from build123d import *

# Parameters (mm, degrees)
F0_W            = 307.8816831112
F0_H            = 200.2553716302
F1_DEPTH        = 25.4
F2_W            = 307.8816831112
F2_H            = 25.4
F3_DEPTH        = 174.76264
F4_DEPTH        = 949.00905
F5_W            = 1324.0270616302
F5_H            = 25.4
F6_DEPTH        = 25.4
F7_W            = 25.4
F7_H            = 1324.0270616302
F8_DEPTH        = 88.17008
F10_D           = 12.7
F10_CSINK_D     = 25.4
F10_CSINK_ANGLE = 90
F12_D           = 12.7
F13_D           = 17.78
F14_D           = 25.4
F15_DEPTH       = 25.4


with BuildPart() as f1:
    # F0 (on Top) → F1 (new body)
    with BuildSketch(Plane.XY):
        with Locations((-0.1046210527, -15.8108584583)):
            Rectangle(F0_W, F0_H)
    extrude(amount=F1_DEPTH)

    # F2 (on face) → F3 (join)
    with BuildSketch(Plane(origin=(0, 84.3168273568, 0), x_dir=(-1, 0, 0), z_dir=(0, 1, 0))):
        with Locations((0.1046210527, 12.7)):
            Rectangle(F2_W, F2_H)
    extrude(amount=F3_DEPTH)

    # F4 (add): a face of the model
    f4_faces = [f1.faces().sort_by_distance(p)[0] for p in [
        (-0.1046210527, 259.0794673568, 12.7),
    ]]
    extrude(f4_faces, amount=F4_DEPTH)

    # F5 (on face) → F6 (join)
    with BuildSketch(Plane(origin=(-154.0454626083, 0, 0), x_dir=(0, -1, 0), z_dir=(-1, 0, 0))):
        with Locations((-546.0749865417, 12.7)):
            Rectangle(F5_W, F5_H)
    extrude(amount=F6_DEPTH)

    # F7 (on face) → F8 (join)
    with BuildSketch(Plane.XY.offset(25.4)):
        with Locations((-166.7454626083, 546.0749865417)):
            Rectangle(F7_W, F7_H)
    extrude(amount=F8_DEPTH)

    # F10 (through all)
    with Locations(Plane.YZ.offset(-154.0454626083)):
        with Locations((0, 71.7426463962), (494.805842638, 71.7426463962), (1091.2485173568, 71.7426463962)):
            CounterSinkHole(F10_D / 2, F10_CSINK_D / 2, counter_sink_angle=F10_CSINK_ANGLE)

    # F12 (through all)
    with Locations(Plane.XY.offset(25.4)):
        with Locations((-35.56, 21.0037976503), (0, 21.0037976503), (40.685325861, 21.0037976503), (79.7552913427, 21.0037976503), (111.532188952, 21.0037976503)):
            Hole(F12_D / 2)

    # F13 (through all)
    with Locations(Plane.XY.offset(25.4)):
        with Locations((-35.56, -10.2521730587), (0, -10.2521730587), (40.685325861, -10.2521730587), (79.7552913427, -10.2521730587), (111.532188952, -10.2521730587)):
            Hole(F13_D / 2)

    # F14 (through all)
    with Locations(Plane.XY.offset(25.4)):
        with Locations((-35.56, -49.8430728912), (19.8480077088, -49.8430728912), (70.3785046935, -49.8430728912), (119.8671087623, -49.8430728912)):
            Hole(F14_D / 2)

    # F11 (on face) → F15 (cut)
    with BuildSketch(Plane.XY.offset(25.4)):
        with BuildLine():
            Line((-130.6297034025, 27.7527463882), (-130.6297034025, 4.3339463882))
            ThreePointArc((-130.6297034025, 4.3339463882), (-118.4733323753, -7.822424639), (-106.3169613481, 4.3339463882))
            Line((-106.3169613481, 4.3339463882), (-106.3169613481, 27.7527463882))
            ThreePointArc((-106.3169613481, 27.7527463882), (-118.4733323753, 39.9091174154), (-130.6297034025, 27.7527463882))
        make_face()
        with BuildLine():
            ThreePointArc((-106.3169613481, -43.5644686222), (-118.4733323753, -31.408097595), (-130.6297034025, -43.5644686222))
            Line((-130.6297034025, -43.5644686222), (-130.6297034025, -63.3748397231))
            Line((-130.6297034025, -63.3748397231), (-130.6297034025, -66.9767335057))
            ThreePointArc((-130.6297034025, -66.9767335057), (-118.4733323753, -79.133104533), (-106.3169613481, -66.9767335057))
            Line((-106.3169613481, -66.9767335057), (-106.3169613481, -43.5644686222))
        make_face()
    extrude(amount=-F15_DEPTH, mode=Mode.SUBTRACT)


solid = f1.part
Work out the finished part from the listing and answer in its coordinate system (mm). A direction names the side the tool comes from. Give positions to 0.01 mm unless a question says otherwise; leave off trailing zeros. Order: outer loops, then holes, each group sorted by start corner. A loop starts at its lowest first (then second) coordinate and runs counter-clockwise, first axis right, second up. Notation, with made-up numbers: M -7.75,56.5 L 36.25,56.5 A23 cw 36.25,77.5 Z; hole C 45,72 d3. An arc over 180 degrees is marked long. Return JSON: item names as keys, results as strings.
Q1. Find the intervals of material crossed by line 1 along Y through (x, z) = (0, 16.25); line 2 along Y through (x, z) = (78, 24); line 3 along X through (y, z) = (513, 35), in increasing order. Write a range as [from, to].
Answer below:
{"line 1": "y = [-115.94, -19.14], [-1.36, 14.65], [27.35, 1208.09]", "line 2": "y = [-115.94, -60], [-39.68, -18.97], [-1.54, 14.9], [27.11, 1208.09]", "line 3": "x = [-179.45, -154.05]"}
Q2. Which of the six approach directions +Z, -Z, +X, -X, +Y, -Y give full straight-line access (tool end or side, diameter ignored) to faces 4 (the face through (-167, 555, 113.57)), 5 (the face through (-106.317, -55, 13))?
Answer below:
{"face 4": "+Z, +X, -X, +Y, -Y", "face 5": "+Z, -Z"}
Q3. Find section A-A, the plane y = 972.5. Write down the section's boundary in (x, z), and give its area (3 significant figures).
Answer below:
{"outline": "M -179.45,0 L 153.84,0 L 153.84,25.4 L -154.05,25.4 L -154.05,113.57 L -179.45,113.57 Z", "area": "10,700 mm^2"}
Q4. Each of these flat-tipped pins is pushed along its axis until it touches: pin 1 (12 mm diameter, centred on y = 104.5, z = 100.5, fed in from +X); pin 2 (20.5 mm diameter, centred on y = 494.81, z = 71.74, fed in from +X). Where does it stop, or does it pass through?
Answer below:
{"pin 1": "stops at x = -154.05", "pin 2": "stops at x = -156.49"}
Q5. The mould has two halves that part along Y. Classify faces 1 (the face through (-160.09, 0.87, 78.34)), 2 (the face through (-51, 1208.089, 23)), 3 (the face through (-154.045, 537, 69)): pulls with the +Y half, pulls with the -Y half, needs draft (parallel to the pull), parting line crosses it, or undercut.
Answer below:
{"face 1": "undercut", "face 2": "pulls with the +Y half", "face 3": "needs draft"}
